Source: CAD feature listing. Evaluate the final solid. Frame: model axes, mm. Give positions to 0.01 mm unless a question says otherwise; leave off trailing zeros. Order: outer loops, then holes, each group sorted by start corner. A loop starts at its lowest first (then second) coordinate and runs counter-clockwise, first axis right, second up. Notation, with made-up numbers: M 88.5,42 L 125.5,42 A20 ccw 125.5,71 Z; hole C 45,-2 d10. An arc over 180 degrees is marked long. One line per question, with ' | ' between items. Start each with the question number.
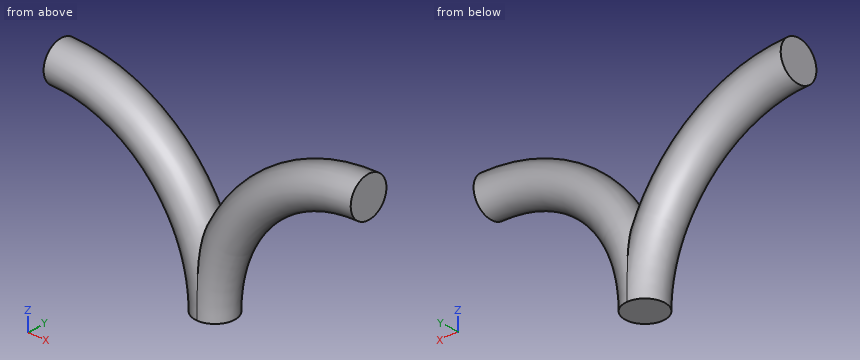
from build123d import *

# Parameters (mm, degrees)
F0_R     = 9.5
F1_ANGLE = 90
F2_W     = 145.696804
F2_H     = 128.937841
F3_DEPTH = 25


with BuildPart() as f1:
    # F0 (on Top) → F1 (revolve)
    with BuildSketch(Plane.XY):
        Circle(F0_R)
    revolve(axis=Axis((74.798293, -7.044435, 0), (0, 1, 0)), revolution_arc=F1_ANGLE)

    # F2 (on Right) → F3 (cut)
    with BuildSketch(Plane.YZ):
        with Locations((-1.890838, 3.012911)):
            Rectangle(F2_W, F2_H)
    extrude(amount=-F3_DEPTH, mode=Mode.SUBTRACT)

    # F4: F1 across plane


with BuildPart() as f1_1:
    add(f1.part)
    add(f1.part.mirror(Plane.YZ))


solid = f1_1.part
Item 1: Line query: line 1 (X direction, y = -3.25, z = 69); line 2 (X direction, y = -1, z = 75); line 3 (Y direction, x = 1, z = 15.5). Output: solid intervals per line, ascending.
Item 2: Pin query (flat end, axial travel): pin 1 Ø4 at (x, z) = (56.5, 58.5) entering from -Y; pin 2 Ø8 at (x, y) = (25, -6.5) entering from +Z; pin 3 Ø4 at (x, z) = (-52.5, 60.5) entering from -Y; pin 4 Ø1 at (y, z) = (6.5, 41.5) entering from +X. Return the tip coordinate at first contact, or that it passes through.
Item 3: Cut plane A-A on y = 1.75. Return the cut outline in (x, z), and give its area (3 significant figures).
Item 4: Cut plane B-B on y = -7. Return the cut outline in (x, z).
Results are:
1) line 1: x = -74.8 to -27.38, 27.38 to 74.8 | line 2: x = -74.8 to -36.43, 36.43 to 74.8 | line 3: y = -9.48 to 9.48
2) pin 1: passes through | pin 2: stops at z = 69.13 | pin 3: stops at y = -4.59 | pin 4: stops at x = 21.78
3) outline: M -74.8,65.46 A65.46 cw -9.34,0 L 9.34,0 A65.46 cw 74.8,65.46 L 74.8,84.14 A84.14 ccw 0,38.52 A84.14 ccw -74.8,84.14 Z | area: 3,900 mm2
4) outline: M -74.8,68.38 A68.38 cw -6.42,0 L 6.42,0 A68.38 cw 74.8,68.38 L 74.8,81.22 A81.22 ccw 0,31.66 A81.22 ccw -74.8,81.22 Z
